```python
from build123d import *

# Parameters (mm, degrees)
ESBO_O1_R                = 4.1
RESSALTO_EXTRUS_O1_DEPTH = 10
ESBO_O2_W                = 23.5
ESBO_O2_H                = 11
CORTE_EXTRUS_O1_DEPTH    = 219.274311432
FILETE1_R                = 2
ESBO_O4_W                = 190
ESBO_O4_H                = 36.622024969
CORTE_EXTRUS_O3_DEPTH    = 289.339020898
RESSALTO_EXTRUS_O2_DEPTH = 190
FILETE3_R                = 9
CORTE_EXTRUS_O4_DEPTH    = 5.5


with BuildPart() as part:
    # Esbo_o1 → Ressalto-extrus_o1 (new, symmetric)
    with BuildSketch(Plane.XY):
        with BuildLine():
            Line((-29.071712183, 188.373872767), (208.88140452, 188.373872767))
            ThreePointArc((208.88140452, 188.373872767), (217.38140452, 179.873872767), (208.88140452, 171.373872767))
            Line((208.88140452, 171.373872767), (-29.071712183, 171.373872767))
            ThreePointArc((-29.071712183, 171.373872767), (-37.571712183, 179.873872767), (-29.071712183, 188.373872767))
        make_face()
        with Locations((-29.071712183, 179.873872767)):
            Circle(ESBO_O1_R, mode=Mode.SUBTRACT)
        with Locations((208.88140452, 179.873872767)):
            Circle(ESBO_O1_R, mode=Mode.SUBTRACT)
    extrude(amount=RESSALTO_EXTRUS_O1_DEPTH, both=True)

    # Esbo_o2 → Corte-extrus_o1 (cut, through all)
    with BuildSketch(Plane(origin=(0, 188.373872767, 0), x_dir=(1, 0, 0), z_dir=(0, 1, 0))):
        with Locations((205.63140452, 0)):
            Rectangle(ESBO_O2_W, ESBO_O2_H)
    extrude(amount=-CORTE_EXTRUS_O1_DEPTH, mode=Mode.SUBTRACT)

    # Filete1
    filete1_edges = [part.edges().sort_by_distance(p)[0] for p in [
        (193.88140452, 179.873872767, -5.5),
        (193.88140452, 179.873872767, 5.5),
    ]]
    fillet(filete1_edges, radius=FILETE1_R)

    # Esbo_o4 → Corte-extrus_o3 (cut, through all)
    with BuildSketch(Plane.XY.offset(10)):
        with Locations((89.904846169, 172.82617811)):
            Rectangle(ESBO_O4_W, ESBO_O4_H)
    extrude(amount=-CORTE_EXTRUS_O3_DEPTH, mode=Mode.SUBTRACT)


with BuildPart() as corte_extrus_o3_piece_1:
    # of the separate pieces the step leaves, piece 1, a body of its own (corte_extrus_o3_pieces)
    add(part.part.solids().sort_by_distance((-5.095153831, 188.373872767, -10))[0])



with BuildPart() as corte_extrus_o3_piece_2:
    # of the separate pieces the step leaves, piece 2, a body of its own (corte_extrus_o3_pieces)
    add(part.part.solids().sort_by_distance((193.88140452, 188.373872767, 3.5))[0])


with BuildPart() as corte_extrus_o3_piece_1_1:
    add(corte_extrus_o3_piece_1.part)

    add(corte_extrus_o3_piece_2.part)  # Ressalto-extrus_o2 merges Corte-extrus_o3 piece 2
    # Esbo_o5 → Ressalto-extrus_o2 (add)
    with BuildSketch(Plane(origin=(-5.095153831, 0, 0), x_dir=(0, 0, -1), z_dir=(1, 0, 0))):
        Polygon((4, 171.373872767), (-4, 171.373872767), (-4, 175.873872767), (-10, 175.873872767), (-10, 183.873872767), (-4, 183.873872767), (-4, 188.373872767), (4, 188.373872767), (4, 183.873872767), (10, 183.873872767), (10, 175.873872767), (4, 175.873872767), align=None)
    extrude(amount=RESSALTO_EXTRUS_O2_DEPTH)

    # Filete3
    # the kernel refuses this fillet: 9 mm, written as the material it adds along each edge
    with BuildSketch(Plane(origin=(-5.095153831, 183.873872767, 10), x_dir=(1, 0, 0), z_dir=(0, 0, -1))) as filete3_piece_1_section:
        with BuildLine():
            CenterArc((7.794228634, -9), FILETE3_R, 90, 60)
            Line((0, -4.5), (-0.155884573, -4.41))
            ThreePointArc((-0.155884573, -4.41), (-0.18, -2.25), (-0.18, 0))
            Line((-0.18, 0), (0, 0.18))
            Line((0, 0.18), (7.794228634, 0.18))
            Line((7.794228634, 0.18), (7.794228634, 0))
        make_face()
    filete3_piece_1 = extrude(amount=25.485571585, mode=Mode.PRIVATE)
    filete3_piece_1 = split(filete3_piece_1, bisect_by=Plane(origin=(-5.095153831, 183.873872767, -10), z_dir=(0, 0, 1)), keep=Keep.TOP, mode=Mode.PRIVATE)
    add(filete3_piece_1)
    with BuildSketch(Plane(origin=(184.904846169, 175.873872767, -15.485571585), x_dir=(0, -1, 0), z_dir=(0, 0, 1))) as filete3_piece_2_section:
        with BuildLine():
            CenterArc((9, -7.794228634), FILETE3_R, 120, 60)
            Line((0, -7.794228634), (-0.18, -7.794228634))
            Line((-0.18, -7.794228634), (-0.18, 0))
            Line((-0.18, 0), (0, 0.18))
            ThreePointArc((0, 0.18), (2.25, 0.18), (4.41, 0.155884573))
            Line((4.41, 0.155884573), (4.5, 0))
        make_face()
    filete3_piece_2 = extrude(amount=25.485571585, mode=Mode.PRIVATE)
    filete3_piece_2 = split(filete3_piece_2, bisect_by=Plane(origin=(184.904846169, 175.873872767, -10), z_dir=(0, 0, 1)), keep=Keep.TOP, mode=Mode.PRIVATE)
    add(filete3_piece_2)
    with BuildSketch(Plane(origin=(184.904846169, 175.873872767, -10), x_dir=(0, -1, 0), z_dir=(0, 0, 1))) as filete3_piece_3_section:
        with BuildLine():
            CenterArc((9, -7.794228634), FILETE3_R, 120, 60)
            Line((0, -7.794228634), (-0.18, -7.794228634))
            Line((-0.18, -7.794228634), (-0.18, 0))
            Line((-0.18, 0), (0, 0.18))
            ThreePointArc((0, 0.18), (2.25, 0.18), (4.41, 0.155884573))
            Line((4.41, 0.155884573), (4.5, 0))
        make_face()
    filete3_piece_3 = extrude(amount=25.485571585, mode=Mode.PRIVATE)
    filete3_piece_3 = split(filete3_piece_3, bisect_by=Plane(origin=(184.904846169, 175.873872767, 10), z_dir=(0, 0, -1)), keep=Keep.TOP, mode=Mode.PRIVATE)
    add(filete3_piece_3)
    with BuildSketch(Plane(origin=(184.904846169, 183.873872767, 10), x_dir=(0, 1, 0), z_dir=(0, 0, -1))) as filete3_piece_4_section:
        with BuildLine():
            CenterArc((9, -7.794228634), FILETE3_R, 120, 60)
            Line((0, -7.794228634), (-0.18, -7.794228634))
            Line((-0.18, -7.794228634), (-0.18, 0))
            Line((-0.18, 0), (0, 0.18))
            ThreePointArc((0, 0.18), (2.25, 0.18), (4.41, 0.155884573))
            Line((4.41, 0.155884573), (4.5, 0))
        make_face()
    filete3_piece_4 = extrude(amount=25.485571585, mode=Mode.PRIVATE)
    filete3_piece_4 = split(filete3_piece_4, bisect_by=Plane(origin=(184.904846169, 183.873872767, -10), z_dir=(0, 0, 1)), keep=Keep.TOP, mode=Mode.PRIVATE)
    add(filete3_piece_4)
    with BuildSketch(Plane(origin=(184.904846169, 183.873872767, 15.485571585), x_dir=(0, 1, 0), z_dir=(0, 0, -1))) as filete3_piece_5_section:
        with BuildLine():
            CenterArc((9, -7.794228634), FILETE3_R, 120, 60)
            Line((0, -7.794228634), (-0.18, -7.794228634))
            Line((-0.18, -7.794228634), (-0.18, 0))
            Line((-0.18, 0), (0, 0.18))
            ThreePointArc((0, 0.18), (2.25, 0.18), (4.41, 0.155884573))
            Line((4.41, 0.155884573), (4.5, 0))
        make_face()
    filete3_piece_5 = extrude(amount=25.485571585, mode=Mode.PRIVATE)
    filete3_piece_5 = split(filete3_piece_5, bisect_by=Plane(origin=(184.904846169, 183.873872767, 10), z_dir=(0, 0, -1)), keep=Keep.TOP, mode=Mode.PRIVATE)
    add(filete3_piece_5)
    with BuildSketch(Plane(origin=(-5.095153831, 175.873872767, -10), x_dir=(1, 0, 0), z_dir=(0, 0, 1))) as filete3_piece_6_section:
        with BuildLine():
            CenterArc((7.794228634, -9), FILETE3_R, 90, 60)
            Line((0, -4.5), (-0.155884573, -4.41))
            ThreePointArc((-0.155884573, -4.41), (-0.18, -2.25), (-0.18, 0))
            Line((-0.18, 0), (0, 0.18))
            Line((0, 0.18), (7.794228634, 0.18))
            Line((7.794228634, 0.18), (7.794228634, 0))
        make_face()
    filete3_piece_6 = extrude(amount=25.485571585, mode=Mode.PRIVATE)
    filete3_piece_6 = split(filete3_piece_6, bisect_by=Plane(origin=(-5.095153831, 175.873872767, 10), z_dir=(0, 0, -1)), keep=Keep.TOP, mode=Mode.PRIVATE)
    add(filete3_piece_6)
    with BuildSketch(Plane(origin=(-5.095153831, 183.873872767, 15.485571585), x_dir=(0, 1, 0), z_dir=(0, 0, -1))) as filete3_piece_7_section:
        with BuildLine():
            CenterArc((9, 7.794228634), FILETE3_R, 180, 60)
            Line((0, 7.794228634), (-0.18, 7.794228634))
            Line((-0.18, 7.794228634), (-0.18, 0))
            Line((-0.18, 0), (0, -0.18))
            ThreePointArc((0, -0.18), (2.25, -0.18), (4.41, -0.155884573))
            Line((4.41, -0.155884573), (4.5, 0))
        make_face()
    filete3_piece_7 = extrude(amount=25.485571585, mode=Mode.PRIVATE)
    filete3_piece_7 = split(filete3_piece_7, bisect_by=Plane(origin=(-5.095153831, 183.873872767, 10), z_dir=(0, 0, -1)), keep=Keep.TOP, mode=Mode.PRIVATE)
    add(filete3_piece_7)
    with BuildSketch(Plane(origin=(-5.095153831, 175.873872767, -15.485571585), x_dir=(1, 0, 0), z_dir=(0, 0, 1))) as filete3_piece_8_section:
        with BuildLine():
            CenterArc((7.794228634, -9), FILETE3_R, 90, 60)
            Line((0, -4.5), (-0.155884573, -4.41))
            ThreePointArc((-0.155884573, -4.41), (-0.18, -2.25), (-0.18, 0))
            Line((-0.18, 0), (0, 0.18))
            Line((0, 0.18), (7.794228634, 0.18))
            Line((7.794228634, 0.18), (7.794228634, 0))
        make_face()
    filete3_piece_8 = extrude(amount=25.485571585, mode=Mode.PRIVATE)
    filete3_piece_8 = split(filete3_piece_8, bisect_by=Plane(origin=(-5.095153831, 175.873872767, -10), z_dir=(0, 0, 1)), keep=Keep.TOP, mode=Mode.PRIVATE)
    add(filete3_piece_8)

    # Esbo_o6 → Corte-extrus_o4 (cut, symmetric)
    with BuildSketch(Plane.XY):
        Polygon((208.88140452, 179.873872767), (196.38140452, 179.873872767), (187.88140452, 188.373872767), (187.88140452, 194.300401894), (208.88140452, 194.300401894), align=None)
    corte_extrus_o4 = extrude(amount=CORTE_EXTRUS_O4_DEPTH, both=True, mode=Mode.SUBTRACT)

    # Espelhar1: Corte-extrus_o4 across plane
    add(corte_extrus_o4.mirror(Plane.ZX.offset(179.873872767)), mode=Mode.SUBTRACT)


solid = corte_extrus_o3_piece_1_1.part
```
Here's how the part is built. I have some questions about the finished solid (model axes, mm). A direction names the side the tool comes from. Coordinates: 2 decimals unless noted, no trailing zeros. Loops run counter-clockwise (first coordinate to the right, second up) from the corner with the lowest first, then second, coordinate; pieces in that order, holes last. Notation, with made-up numbers: M 75.5,57 L 92.5,57 A28 ccw 92.5,89 Z; hole C 7.25,73 d3. An arc over 180 degrees is marked long. One line per item, written item: value.
1. Thinking about a two-plate mould opening in Y: for faces 6 (the flat face through (203, 180, 5.5)), 7 (the cylindrical face through (-27.18, 176.236, -0.14)), 8 (the cylindrical face through (-1.744, 185.047, -6.958)), which applies, +Y half, -Y half, draft (parallel to the pull), parting line (faces both ways), or undercut?
Geometry says:
face 6: draft
face 7: undercut
face 8: +Y half
2. Will these pins go through, and if not, where does the flat tip stop? pin 1 Ø5 at (x, z) = (95.5, 5) entering from +Y; pin 2 Ø5 at (x, y) = (109, 172.5) entering from -Z; pin 3 Ø3 at (x, z) = (112, 7.5) entering from +Y; pin 4 Ø2 at (y, z) = (181.5, 7.5) entering from -X.
Geometry says:
pin 1: stops at y = 188.37
pin 2: stops at z = -4
pin 3: stops at y = 183.87
pin 4: stops at x = -37.55
3. Imagine slicing it at B-B (z = -1). List the corners of the cut face in (x, y) for me.
Geometry says:
outline: M -29.07,171.37 L 187.88,171.37 L 193.88,177.37 L 193.88,182.37 L 187.88,188.37 L -29.07,188.37 A8.5 ccw Z; hole C -29.07,179.87 d8.2
4. Please list where these lines run through material, in increasing order: probe 1 along Z at (x, y) = (196, 180); probe 2 along X at (y, z) = (181.5, 8.25); probe 3 along Y at (x, z) = (11, -5).
Geometry says:
probe 1: z = -10 to -5.5, 5.5 to 10
probe 2: x = -37.41 to -32.84, -25.31 to 205.12, 212.65 to 217.22
probe 3: y = 175.87 to 183.87
5. On a 3-axis mill with a long thin cutter (end or side, diameter ignored), from which of +Z, -Z, +X, -X, +Y, -Y can I reach the whole of each face in a straight line? I mean faces 1 (the flat face through (89, 183.874, -7)), 2 (the cylindrical face through (-1.744, 174.701, -7.042)), 3 (the flat face through (193.881, 180, 0)), 4 (the cylindrical face through (-1.744, 185.047, 7.042)), 5 (the cylindrical face through (-1.744, 174.701, 6.958)). Say none if no direction works.
Geometry says:
face 1: -Z, +Y
face 2: -Z, -Y
face 3: +X, +Y, -Y
face 4: +Z, +Y
face 5: +Z, -Y
6. Imagine slicing it at A-A (x = 70). List the corners of the cut face in (y, z) for me.
Geometry says:
outline: M 171.37,-4 L 175.87,-4 L 175.87,-10 L 183.87,-10 L 183.87,-4 L 188.37,-4 L 188.37,4 L 183.87,4 L 183.87,10 L 175.87,10 L 175.87,4 L 171.37,4 Z
